Source: CAD feature listing. Evaluate the final solid. Frame: model axes, mm. Give positions to 0.01 mm unless a question says otherwise; leave off trailing zeros. Write each loop counter-clockwise with the first axis right and the second up, starting at its lowest first coordinate (ties: lowest second). Pieces come first, ordered by that corner, then holes. Notation, with made-up numbers: (34.5, 22) - (68.5, 22) arc R24 cw to (68.5, 61) - close; hole circle Ø4 at (-38, 23). An arc over 180 degrees is marked (long way). One line per question, with ' | ' between items. Start each with the question number.
(1) Pin query (flat end, axial travel): pin 1 (4 mm diameter, centred on x = -14.33, z = 5.33, fed in from -Y); pin 2 (2 mm diameter, centred on x = 7.5, z = 6, fed in from -Y); pin 3 (5 mm diameter, centred on x = -30, z = 3, fed in from +Y); pin 4 (3.5 mm diameter, centred on y = -59.5, z = 4, fed in from +X). Return the tip coordinate at first contact, or that it passes through.
(2) Section A-A, the plane x = -10. Return loops of the section in (y, z), plus the area to 3 significant figures.
(3) Section D-D, the plane y = 5. Return loops of the section in (x, z), plus the area to 3 significant figures.
(4) Section B-B, the plane x = 12. Return loops of the section in (y, z).
(5) Ray query, line 1 (Y direction, x = 29.5, z = 8); line 2 (Y direction, x = -28, z = 6). Return the intervals inside material, ascending. Write a range as [from, to].
(6) Section C-C, the plane y = 24. Return loops of the section in (x, z).
```python
from build123d import *

# Parameters (mm, degrees)
F1_DEPTH  = 9.652
F2_T      = -0.127
F3_W      = 10.16
F3_H      = 3.048
F3_R      = 2.54
F4_DEPTH  = 4.572
F5_W      = 29.768799
F5_H      = 6.858
F6_DEPTH  = 4.572
F7_W      = 44.958
F7_H      = 7.4676
F8_DEPTH  = 4.572
F9_R      = 8.497621
F10_DEPTH = 25.4


with BuildPart() as f1:
    # F0 (on Top) → F1 (new body)
    with BuildSketch(Plane.XY):
        with BuildLine():
            Line((22.479, 60.96), (-22.479, 60.96))
            ThreePointArc((-22.479, 60.96), (-29.663205, 57.984205), (-32.639, 50.8))
            Line((-32.639, 50.8), (-32.639, -50.8))
            ThreePointArc((-32.639, -50.8), (-29.663205, -57.984205), (-22.479, -60.96))
            Line((-22.479, -60.96), (22.479, -60.96))
            ThreePointArc((22.479, -60.96), (29.663205, -57.984205), (32.639, -50.8))
            Line((32.639, -50.8), (32.639, 50.8))
            ThreePointArc((32.639, 50.8), (29.663205, 57.984205), (22.479, 60.96))
        make_face()
    extrude(amount=F1_DEPTH)

    # F2
    f2_openings = [f1.faces().sort_by_distance(p)[0] for p in [
        (0, 0, 9.652),
    ]]
    offset(amount=F2_T, openings=f2_openings)

    # F3 (on face) → F4 (cut)
    with BuildSketch(Plane.XZ.offset(-60.833)):
        with Locations((15.544799, 5.9436)):
            Rectangle(F3_W, F3_H)
        with Locations((-14.3256, 5.334001)):
            Circle(F3_R)
    extrude(amount=-F4_DEPTH, mode=Mode.SUBTRACT)

    # F5 (on face) → F6 (cut)
    with BuildSketch(Plane(origin=(-32.639, 0, 0), x_dir=(0, -1, 0), z_dir=(-1, 0, 0))):
        with Locations((-35.9156, 3.429)):
            Rectangle(F5_W, F5_H)
    extrude(amount=-F6_DEPTH, mode=Mode.SUBTRACT)

    # F7 (on face) → F8 (cut)
    with BuildSketch(Plane.XZ.offset(60.96)):
        with Locations((0, 3.7338)):
            Rectangle(F7_W, F7_H)
    extrude(amount=-F8_DEPTH, mode=Mode.SUBTRACT)

    # F9 (on face) → F10 (cut)
    with BuildSketch(Plane(origin=(0, 0, 0), x_dir=(1, 0, 0), z_dir=(0, 0, -1))):
        with Locations((22.479, -50.8)):
            Circle(F9_R)
    extrude(amount=-F10_DEPTH, mode=Mode.SUBTRACT)


solid = f1.part
```
Check sheet entries:
1) pin 1: through | pin 2: y = 60.83 | pin 3: y = 59.63 | pin 4: x = 29.89
2) outline: (-60.96, 7.47) - (-60.83, 7.47) - (-60.83, 9.65) - (-60.96, 9.65) - close; (-56.39, 0) - (60.96, 0) - (60.96, 9.65) - (60.83, 9.65) - (60.83, 0.13) - (-56.39, 0.13) - close | area: 16.4 mm²
3) outline: (-32.64, 0) - (32.64, 0) - (32.64, 9.65) - (32.51, 9.65) - (32.51, 0.13) - (-32.51, 0.13) - (-32.51, 9.65) - (-32.64, 9.65) - close | area: 10.7 mm²
4) outline: (-60.96, 7.47) - (-60.83, 7.47) - (-60.83, 9.65) - (-60.96, 9.65) - close; (-56.39, 0) - (60.96, 0) - (60.96, 4.42) - (60.83, 4.42) - (60.83, 0.13) - (-56.39, 0.13) - close; (60.83, 7.47) - (60.96, 7.47) - (60.96, 9.65) - (60.83, 9.65) - close
5) line 1: [-58.14, -57.97], [57.97, 58.14] | line 2: [-59.33, -59.18], [59.18, 59.33]
6) outline: (-32.64, 6.86) - (-32.51, 6.86) - (-32.51, 9.65) - (-32.64, 9.65) - close; (-28.07, 0) - (32.64, 0) - (32.64, 9.65) - (32.51, 9.65) - (32.51, 0.13) - (-28.07, 0.13) - close
